from build123d import *

# Parameters (mm, degrees)
F1_DEPTH = 8.5
F3_START = 2
F2_W     = 17
F2_H     = 3.2842862599
F3_DEPTH = 4.5


with BuildPart() as f1:
    # F0 (on Top) → F1 (new body)
    with BuildSketch(Plane.XY):
        Polygon((-27, 0), (0, 0), (-10, 10), (-27, 10), align=None)
        Polygon((-27, -7), (0, 0), (-27, 0), align=None)
        Polygon((-10, 10), (0, 0), (2.8284271247, 0), (-10.0005280692, 12.828955194), align=None)
        Polygon((-27, 10), (-10, 10), (-10.0005280692, 12.828955194), (-27, 12.8257819737), align=None)
    extrude(amount=F1_DEPTH)

    # F2 (on Top) → F3 (cut)
    with BuildSketch(Plane.XY.offset(F3_START)):
        Polygon((-27, -7), (0, 0), (-27, 0), align=None)
        Polygon((-27, 0), (0, 0), (-10, 10), (-27, 10), align=None)
        with Locations((-18.5, 11.6421431299)):
            Rectangle(F2_W, F2_H)
    extrude(amount=F3_DEPTH, mode=Mode.SUBTRACT)


solid = f1.part
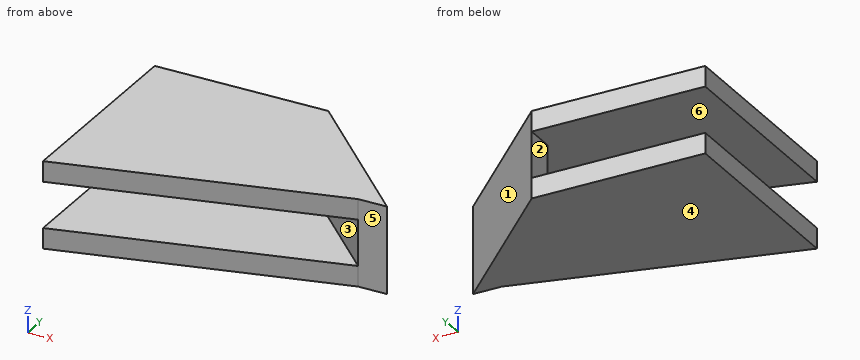
Design review of the part built by this model. Coordinates are the model's own, in mm. Face numbers are marked on the shaded views. A direction names the side the tool comes from. Round coordinates to 2 decimals unless told otherwise and drop trailing zeros. Write each loop counter-clockwise with the first axis right and the second up, starting at its lowest first coordinate (ties: lowest second). Pieces come first, ordered by that corner, then holes. Notation, with made-up numbers: M -10.75,-34 L 41.25,-34 A18 cw 41.25,-22 Z; hole C -10,30.5 d9. An arc over 180 degrees is marked long. One line per item, written item: value. Start each with the question number.
1. To check wall thickness, follow probe 1 along Z at (x, y) = (-5, -0.5); probe 2 along Y at (x, z) = (-16, 0.5); probe 3 along Y at (x, z) = (-1.5, 5.5). State the ranges of each line that lie inside material, in increasing order. Write a range as from..to.
2. Take a section at D-D on y = 11.5. State the section outline as (x, z) points, then the cut area to 3 significant figures.
3. Take a section at A-A on y = -2.5. State the section outline as (x, z) points, then the cut area to 3 significant figures.
4. Take a section at C-C on z = 1.5. State the section outline as (x, y) points, then the cut area to 3 significant figures.
5. For the marked faces 1, 2 and 3, list the 3-axis set-ups (+Z, -Z, +X, -X, +Y, -Y) from which the entire face can be reached by the end or side of a thin tool; tool diameter is ignored.
6. Draft analysis for pull direction Z (two halves, no side actions). For the marked faces 4, 5 and 6, state which applies: pulls with the +Z half, pulls with the -Z half, needs draft (parallel to the pull), parting line crosses it, or undercut.
7. Clearance check with flat-ended pins moving along their axes: P1, Ø5, axis at y = 4.5, z = 3.5, coming from the +X side; P2, Ø4, axis at y = 6, z = 4.5, coming from the +X side; P3, Ø1, axis at x = -8, z = 4.5, coming from the -Y side. State where each tip first meets the part, or that it passes through.
8. Take a section at B-B on x = -15.25. State the section outline as (y, z) points, then the cut area to 3 significant figures.
Computed:
1. probe 1: z = 0..2, 6.5..8.5
1. probe 2: y = -4.15..12.83
1. probe 3: y = 1.5..4.33
2. outline: M -27,0 L -8.67,0 L -8.67,8.5 L -27,8.5 L -27,6.5 L -10,6.5 L -10,2 L -27,2 Z
2. area: 79.3 mm²
3. outline: M -27,0 L -9.64,0 L -9.64,2 L -27,2 Z; M -27,6.5 L -9.64,6.5 L -9.64,8.5 L -27,8.5 Z
3. area: 69.4 mm²
4. outline: M -27,-7 L 0,0 L 2.83,0 L -10,12.83 L -27,12.83 Z
4. area: 395 mm²
5. face 1: +Z, -Z, +X, +Y
5. face 2: -X, +Y, -Y
5. face 3: -X, -Y
6. face 4: pulls with the -Z half
6. face 5: needs draft
6. face 6: undercut
7. P1: stops at x = 0.83
7. P2: stops at x = -1.17
7. P3: stops at y = 7.5
8. outline: M -3.95,0 L 12.83,0 L 12.83,2 L -3.95,2 Z; M -3.95,6.5 L 12.83,6.5 L 12.83,8.5 L -3.95,8.5 Z
8. area: 67.1 mm²
